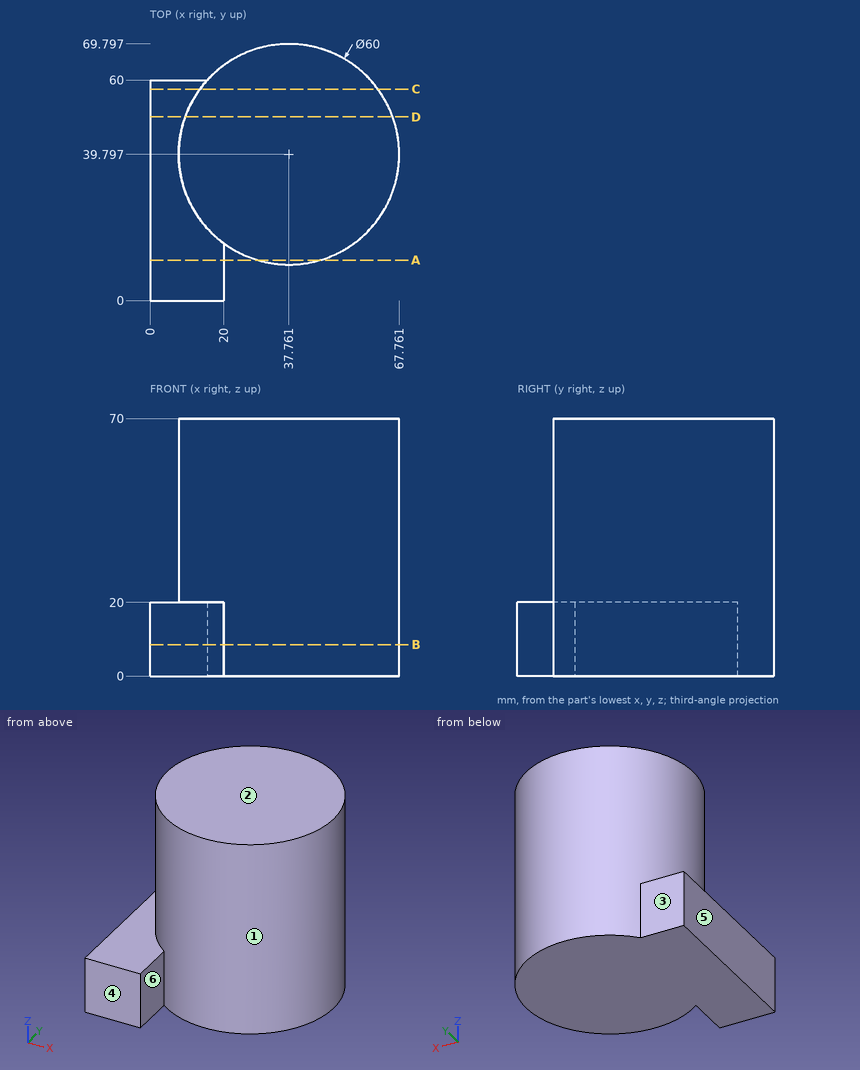
Verification items for this drawing (mm, ordinates from the low corner). A direction names the side the tool comes from. Coordinates: 2 decimals unless noted, no trailing zeros. Order: outer loops, then holes, each group sorted by start corner. A loop starts at its lowest first (then second) coordinate and runs counter-clockwise, first axis right, second up. Notation, with made-up numbers: (43, 10.25) - (48, 10.25) arc R22 cw to (48, 46.25) - close; hole circle Ø9 at (60, 5). An arc over 180 degrees is marked (long way). Answer as a JSON object with one key per item and string values. Group by question number.
Item 1: Sectioned sample at C-C, the plane y = 57.5. Record the cut outline in (x, z).
Item 2: Sectioned sample at A-A, the plane y = 11. Record the cut outline in (x, z), and give its area (3 significant figures).
Item 3: Sectioned sample at D-D, the plane y = 50. Record the cut outline in (x, z), and give its area (3 significant figures).
Item 4: Depth check by flat-ended pin: pin 1 Ø4 at (x, z) = (8, 16.5) entering from +Y; pin 2 Ø12 at (x, z) = (47, 47.5) entering from +Y; pin 3 Ø17 at (x, z) = (10, 11.5) entering from +Y. Enter the tip coordinate at first touch or a pass-through.
Item 5: Tool access check on the marked faces 1, 2 and 3. Record the directions out of +Z, -Z, +X, -X, +Y, -Y that give a thin tool (end or side, any length) a straight path to the whole face; none if there is none.
Item 6: Sectioned sample at B-B, the plane z = 8.5. Record the cut outline in (x, y), and give its area (3 significant figures).
Item 7: Scan lines: probe 1 along Z at (x, y) = (13.5, 18.5); probe 2 along Y at (x, z) = (14, 10). Record each from-to range of solid material in increasing order.
Item 8: Draft check along X on the marked faces 4, 5 and 6. Enter one of: +X half, -X half, draft (parallel to the pull), parting line (faces both ways), or undercut.
Resolved:
{
 "1": {"outline": "(0, 0) - (61.98, 0) - (61.98, 70) - (13.54, 70) - (13.54, 20) - (0, 20) - close"},
 "2": {"outline": "(0, 0) - (20, 0) - (20, 20) - (0, 20) - close; (29.35, 0) - (46.17, 0) - (46.17, 70) - (29.35, 70) - close", "area": "1,580 mm^2"},
 "3": {"outline": "(0, 0) - (65.97, 0) - (65.97, 70) - (9.55, 70) - (9.55, 20) - (0, 20) - close", "area": "4,140 mm^2"},
 "4": {"pin 1": "y = 60", "pin 2": "y = 69.62", "pin 3": "y = 62.8"},
 "5": {"face 1": "+Z", "face 2": "+Z, +X, -X, +Y, -Y", "face 3": "+Z, -Z, -X, +Y"},
 "6": {"outline": "(0, 0) - (20, 0) - (20, 15.62) arc R30 ccw (long way) to (15.58, 60) - (0, 60) - close", "area": "3,620 mm^2"},
 "7": {"probe 1": "0 to 20", "probe 2": "0 to 60"},
 "8": {"face 4": "draft", "face 5": "-X half", "face 6": "undercut"}
}
